from build123d import *

# Parameters (mm, degrees)
F0_R     = 4.7625
F0_R_2   = 66.675
F0_R_3   = 2.032
F0_R_4   = 6.35
F0_R_5   = 2.0193
F0_R_6   = 1.5875
F1_DEPTH = 2.286
F2_R     = 5.08
F3_R     = 5.08
F4_R     = 4.0005
F5_DEPTH = 25.4


with BuildPart() as f1:
    # F0 (on Top) → F1 (new body)
    with BuildSketch(Plane.XY):
        with BuildLine():
            ThreePointArc((79.375, 0), (0, 79.375), (-79.375, 0))
            ThreePointArc((-79.375, 0), (-65.703381, -44.536011), (-29.398148, -73.73018))
            ThreePointArc((-29.398148, -73.73018), (0, -79.375), (29.398148, -73.73018))
            ThreePointArc((29.398148, -73.73018), (65.703381, -44.536011), (79.375, 0))
        make_face()
        with Locations((-36.572162, -63.344843)):
            Circle(F0_R, mode=Mode.SUBTRACT)
        with Locations((-73.144324, 0)):
            Circle(F0_R, mode=Mode.SUBTRACT)
        with Locations((36.572162, -63.344843)):
            Circle(F0_R, mode=Mode.SUBTRACT)
        Circle(F0_R_2, mode=Mode.SUBTRACT)
        with Locations((73.144324, 0)):
            Circle(F0_R, mode=Mode.SUBTRACT)
        with Locations((-36.572162, 63.344843)):
            Circle(F0_R, mode=Mode.SUBTRACT)
        with Locations((36.572162, 63.344843)):
            Circle(F0_R, mode=Mode.SUBTRACT)
        with BuildLine():
            Line((-79.375, 152.4), (-79.375, 0))
            ThreePointArc((-79.375, 0), (0, 79.375), (79.375, 0))
            Line((79.375, 0), (79.375, 152.4))
            Line((79.375, 152.4), (-79.375, 152.4))
        make_face()
        with Locations((-25.4, 127)):
            Circle(F0_R_3, mode=Mode.SUBTRACT)
        with Locations((0, 127)):
            Circle(F0_R_4, mode=Mode.SUBTRACT)
        with Locations((25.4, 127)):
            Circle(F0_R_5, mode=Mode.SUBTRACT)
        with BuildLine():
            ThreePointArc((29.398148, -73.73018), (0, -79.375), (-29.398148, -73.73018))
            ThreePointArc((-29.398148, -73.73018), (-26.493729, -76.065714), (-25.4, -79.628595))
            Line((-25.4, -79.628595), (-25.4, -104.775))
            Line((-25.4, -104.775), (0, -104.775))
            Line((0, -104.775), (25.4, -104.775))
            Line((25.4, -104.775), (25.4, -79.628595))
            ThreePointArc((25.4, -79.628595), (26.493729, -76.065714), (29.398148, -73.73018))
        make_face()
        with Locations((-21.401391, -92.075)):
            Circle(F0_R_6, mode=Mode.SUBTRACT)
        with Locations((0, -92.075)):
            Circle(F0_R_6, mode=Mode.SUBTRACT)
        with Locations((22.656089, -92.075)):
            Circle(F0_R_6, mode=Mode.SUBTRACT)
    extrude(amount=F1_DEPTH)

    # F2
    f2_edges = [f1.edges().sort_by_distance(p)[0] for p in [
        (-79.375, 152.4, 1.143),
        (79.375, 152.4, 1.143),
    ]]
    fillet(f2_edges, radius=F2_R)

    # F3
    f3_edges = [f1.edges().sort_by_distance(p)[0] for p in [
        (25.4, -104.775, 1.143),
        (-25.4, -104.775, 1.143),
    ]]
    fillet(f3_edges, radius=F3_R)

    # F4 (on face) → F5 (join)
    with BuildSketch(Plane.XY.offset(2.286)):
        with Locations((-31.75, 101.6)):
            Circle(F4_R)
        with Locations((31.75, 101.6)):
            Circle(F4_R)
    extrude(amount=F5_DEPTH)


solid = f1.part
The listing builds one solid part. Answer for the finished solid, in the listing's coordinates (mm). A direction names the side the tool comes from. Round coordinates to 2 decimals unless told otherwise and drop trailing zeros. Write each loop counter-clockwise with the first axis right and the second up, starting at its lowest first coordinate (ties: lowest second). Pieces come first, ordered by that corner, then holes. Notation, with made-up numbers: M 14,-3 L 44,-3 A23 ccw 44,28 Z; hole C 24,71.5 d11. An arc over 180 degrees is marked long. Write each question's results on one line, items separated by ' | '. Start each with the question number.
Item 1: Straight lines are drawn through the part: L1, parallel to Z at x = -21.5, y = 64.5; L2, parallel to X at y = 103, z = 9.25. For each, find the intervals that lie inside material, in ascending order. Write a range as [from, to].
Item 2: For a pull along Y with two mould halves and no side action, classify faces 1 (the face through (-37.192, -58.623, 1.127)), 2 (the face through (-32, 102, 27.686)), 3 (the face through (-77.85, 150.95, 1.16)) as pulls with the +Y half, pulls with the -Y half, needs draft (parallel to the pull), parting line crosses it, or undercut.
Item 3: Flat-ended cylindrical pins translate along their axes: pin 1 Ø2.5 at (x, y) = (0, -92.075) entering from -Z; pin 2 Ø12.5 at (x, y) = (73.14, 0) entering from +Z; pin 3 Ø5 at (x, z) = (30, 9.5) entering from +Y; pin 4 Ø10 at (x, z) = (-34.5, 22.5) entering from -Y. Find the tip coordinate at first contact, or state that the pin passes through.
Item 4: A cutting plane is placed at C-C on y = 101.6. Write down the section's boundary in (x, z) (1 decimal), and give its area (3 significant figures).
Item 5: A cutting plane is placed at D-D on z = 8. Write down the section's boundary in (x, y).
Item 6: For faces 4 (the face through (-34.7, 104.3, 14.8)), 5 (the face through (-77.902, 0.209, 1.127)), determine the directions among +Z, -Z, +X, -X, +Y, -Y from which every point of the face is accessible in a straight line to the end or side of a thin tool.
Item 7: A cutting plane is placed at A-A on y = 46.5. Write down the section's boundary in (x, z) (3 decimals).
Item 8: A cutting plane is placed at B-B on x = 62.5. Write down the section's boundary in (y, z).
Check sheet entries:
1) L1: [0, 2.29] | L2: [-35.5, -28], [28, 35.5]
2) face 1: undercut | face 2: needs draft | face 3: pulls with the +Y half
3) pin 1: through | pin 2: z = 2.29 | pin 3: y = 105.6 | pin 4: y = 97.6
4) outline: M -79.4,0 L 79.4,0 L 79.4,2.3 L 35.8,2.3 L 35.8,27.7 L 27.7,27.7 L 27.7,2.3 L -27.7,2.3 L -27.7,27.7 L -35.8,27.7 L -35.8,2.3 L -79.4,2.3 Z | area: 769 mm²
5) outline: C -31.75,101.6 d8; C 31.75,101.6 d8
6) face 4: +Z | face 5: +Z, -Z
7) outline: M -79.375,0 L -47.784,0 L -47.784,2.286 L -79.375,2.286 Z; M 47.784,0 L 79.375,0 L 79.375,2.286 L 47.784,2.286 Z
8) outline: M -48.93,0 L -23.22,0 L -23.22,2.29 L -48.93,2.29 Z; M 23.22,0 L 152.4,0 L 152.4,2.29 L 23.22,2.29 Z
